Source: CAD feature listing. Evaluate the final solid. Frame: model axes, mm. A direction names the side the tool comes from. Give positions to 0.01 mm unless a question says otherwise; leave off trailing zeros. Loops run counter-clockwise (first coordinate to the right, second up) from the corner with the lowest first, then second, coordinate; pieces in that order, holes last. Notation, with made-up numbers: (62, 50) -> (67, 50) arc R23 cw to (67, 70) -> close; hole circle Ø4 at (39.5, -28). An arc over 180 degrees is marked (long way). Return JSON: item names as keys, results as strings. Group by question number.
(1) Cut plane C-C on z = 54. Return loops of the section in (x, y).
(2) Access query for faces 4 (the face through (0, -24, 11)), 5 (the face through (-18.179, -18.113, 36.465)), 6 (the face through (13.1, 13.7, 37)). Directions: +Z, -Z, +X, -X, +Y, -Y. A direction counts if a zero-diameter tool reaches every point of the face in a straight line with its end or side. Return the directions, or none.
(3) Cut plane D-D on z = 64. Return loops of the section in (x, y).
(4) Cut plane A-A on y = 0. Return loops of the section in (x, z).
(5) Draft query along Y for faces 1 (the face through (0, -27, 6)), 2 (the face through (17, -17, 35)), 3 (the face through (18.179, 18.113, 36.465)). Return one class per face: released by +Y, released by -Y, zero draft, split by the parting line, or undercut.
(6) Pin query (flat end, axial travel): pin 1 (1.5 mm diameter, centred on x = -1, z = 37.5, fed in from -Y); pin 2 (3 mm diameter, centred on y = 10, z = 37.5, fed in from -X); pin 3 (2 mm diameter, centred on y = -8.5, z = 54.5, fed in from -X); pin 4 (5 mm diameter, centred on y = 7, z = 70.5, fed in from +X) (1 decimal). Return the tip coordinate at first contact, or that it passes through.
(7) Ray query, line 1 (Y direction, x = 15.5, z = 1.1); line 2 (X direction, y = -15.5, z = 16.5); line 3 (X direction, y = 15, z = 1). Return the intervals inside material, ascending. Write a range as from..to.
```python
from build123d import *

# Parameters (mm, degrees)
F0_W      = 42
F0_H      = 42
F1_DEPTH  = 34
F2_SIZE   = 5
F3_W      = 16
F3_H      = 6
F4_DEPTH  = 11
F5_R      = 0.5
F6_DEPTH  = 5
F7_R      = 1.75
F8_DEPTH  = 39.001
F9_R      = 3
F10_DEPTH = 4
F11_R     = 18
F12_DEPTH = 22
F13_R     = 11
F14_DEPTH = 2
F15_R     = 4
F16_DEPTH = 20
F17_SIZE  = 0.5
F19_DEPTH = 14.75
F20_R     = 1.75
F21_DEPTH = 22
F22_R     = 3
F23_DEPTH = 3
F24_R     = 5
F25_DEPTH = 4


with BuildPart() as f1:
    # F0 (on Top) → F1 (new body)
    with BuildSketch(Plane.XY):
        Rectangle(F0_W, F0_H)
    extrude(amount=F1_DEPTH)

    # F2
    f2_edges = [f1.edges().sort_by_distance(p)[0] for p in [
        (-21, -21, 17),
        (21, -21, 17),
        (21, 21, 17),
        (-21, 21, 17),
    ]]
    chamfer(f2_edges, length=F2_SIZE)

    # F3 (on Top) → F4 (join)
    with BuildSketch(Plane.XY):
        with Locations((0, -24)):
            Rectangle(F3_W, F3_H)
    extrude(amount=F4_DEPTH)

    # F5
    f5_edges = [f1.edges().sort_by_distance(p)[0] for p in [
        (21, 0, 34),
        (18.5, -18.5, 34),
        (18.5, 18.5, 34),
        (0, -21, 34),
        (0, 21, 34),
        (-18.5, -18.5, 34),
        (-18.5, 18.5, 34),
        (-21, 0, 34),
        (21, 0, 0),
        (18.5, 18.5, 0),
        (0, 21, 0),
        (-18.5, 18.5, 0),
        (-21, 0, 0),
        (-18.5, -18.5, 0),
        (-12, -21, 0),
        (-8, -24, 0),
        (0, -27, 0),
        (8, -24, 0),
        (12, -21, 0),
        (18.5, -18.5, 0),
    ]]
    fillet(f5_edges, radius=F5_R)

    # F6 (add): a face of the model
    f6_faces = [f1.faces().sort_by_distance(p)[0] for p in [
        (0, 0, 34),
    ]]
    extrude(f6_faces, amount=F6_DEPTH)

    # F7 (on face) → F8 (cut, through all)
    with BuildSketch(Plane(origin=(0, 0, 0), x_dir=(1, 0, 0), z_dir=(0, 0, -1))):
        with Locations((-15.5, 15.5)):
            Circle(F7_R)
        with Locations((-15.5, -15.5)):
            Circle(F7_R)
        with Locations((15.5, -15.5)):
            Circle(F7_R)
        with Locations((15.5, 15.5)):
            Circle(F7_R)
    extrude(amount=-F8_DEPTH, mode=Mode.SUBTRACT)

    # F9 (on face) → F10 (cut)
    with BuildSketch(Plane.XY.offset(39)):
        with Locations((-15.5, 15.5)):
            Circle(F9_R)
        with Locations((-15.5, -15.5)):
            Circle(F9_R)
        with Locations((15.5, -15.5)):
            Circle(F9_R)
        with Locations((15.5, 15.5)):
            Circle(F9_R)
    extrude(amount=-F10_DEPTH, mode=Mode.SUBTRACT)

    # F11 (on face) → F12 (join)
    with BuildSketch(Plane.XY.offset(39)):
        Circle(F11_R)
    extrude(amount=F12_DEPTH)

    # F13 (on face) → F14 (join)
    with BuildSketch(Plane.XY.offset(61)):
        Circle(F13_R)
    extrude(amount=F14_DEPTH)

    # F15 (on face) → F16 (join)
    with BuildSketch(Plane.XY.offset(61)):
        Circle(F15_R)
    extrude(amount=F16_DEPTH)

    # F17
    f17_edges = [f1.edges().sort_by_distance(p)[0] for p in [
        (-4, 0, 81),
    ]]
    chamfer(f17_edges, length=F17_SIZE)

    # F18 (on face) → F19 (cut)
    with BuildSketch(Plane.XY.offset(81)):
        with BuildLine():
            Line((-2.6457513111, 3), (2.6457513111, 3))
            ThreePointArc((2.6457513111, 3), (0, 4), (-2.6457513111, 3))
        make_face()
    extrude(amount=-F19_DEPTH, mode=Mode.SUBTRACT)

    # F20 (on face) → F21 (cut, through all)
    with BuildSketch(Plane.XY.offset(61)):
        with Locations((-9.8994949366, 9.8994949366)):
            Circle(F20_R)
        with Locations((-9.8994949366, -9.8994949366)):
            Circle(F20_R)
        with Locations((9.8994949366, -9.8994949366)):
            Circle(F20_R)
        with Locations((9.8994949366, 9.8994949366)):
            Circle(F20_R)
    extrude(amount=-F21_DEPTH, mode=Mode.SUBTRACT)

    # F22 (on face) → F23 (cut)
    with BuildSketch(Plane(origin=(0, 0, 0), x_dir=(1, 0, 0), z_dir=(0, 0, -1))):
        with Locations((-15.5, 15.5)):
            Circle(F22_R)
        with Locations((-15.5, -15.5)):
            Circle(F22_R)
        with Locations((15.5, -15.5)):
            Circle(F22_R)
        with Locations((15.5, 15.5)):
            Circle(F22_R)
    extrude(amount=-F23_DEPTH, mode=Mode.SUBTRACT)

    # F24 (on face) → F25 (cut)
    with BuildSketch(Plane(origin=(0, 0, 0), x_dir=(1, 0, 0), z_dir=(0, 0, -1))):
        Circle(F24_R)
    extrude(amount=-F25_DEPTH, mode=Mode.SUBTRACT)


solid = f1.part
```
Answers:
{
 "1": {"outline": "circle Ø36 at (0, 0); hole circle Ø3.5 at (-9.9, -9.9); hole circle Ø3.5 at (-9.9, 9.9); hole circle Ø3.5 at (9.9, -9.9); hole circle Ø3.5 at (9.9, 9.9)"},
 "2": {"face 4": "+Z, +X, -X, -Y", "face 5": "+Z, -X, -Y", "face 6": "+Z"},
 "3": {"outline": "circle Ø8 at (0, 0)"},
 "4": {"outline": "(-21, 0.5) arc R0.5 ccw to (-20.5, 0) -> (-5, 0) -> (-5, 4) -> (5, 4) -> (5, 0) -> (20.5, 0) arc R0.5 ccw to (21, 0.5) -> (21, 33.5) arc R0.5 ccw to (20.5, 34) -> (20.5, 39) -> (18, 39) -> (18, 61) -> (11, 61) -> (11, 63) -> (4, 63) -> (4, 80.5) -> (3.5, 81) -> (-3.5, 81) -> (-4, 80.5) -> (-4, 63) -> (-11, 63) -> (-11, 61) -> (-18, 61) -> (-18, 39) -> (-20.5, 39) -> (-20.5, 34) arc R0.5 ccw to (-21, 33.5) -> close"},
 "5": {"face 1": "released by -Y", "face 2": "undercut", "face 3": "released by +Y"},
 "6": {"pin 1": "y = -20.5", "pin 2": "x = -20.5", "pin 3": "x = -16.36", "pin 4": "through"},
 "7": {"line 1": "-21..-18.5, -12.5..12.5, 18.5..21", "line 2": "-21..-17.25, -13.75..13.75, 17.25..21", "line 3": "-21..-18.46, -12.54..12.54, 18.46..21"}
}
